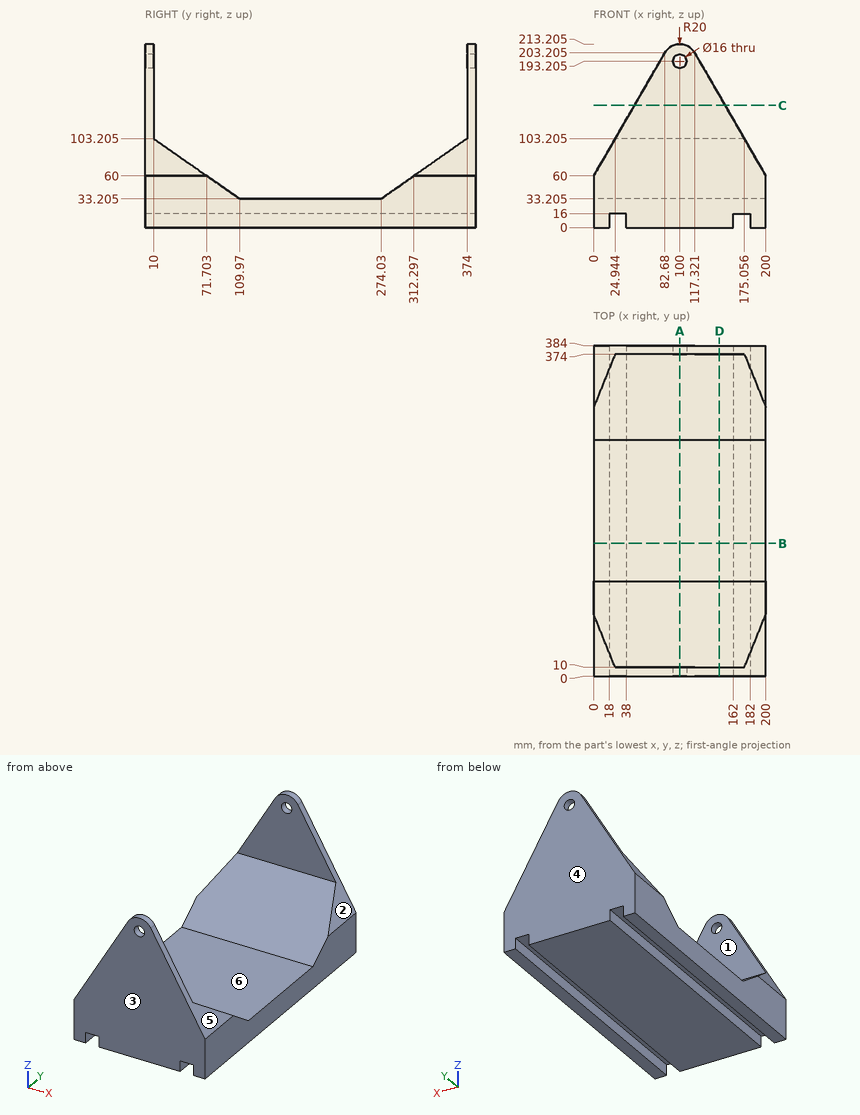
Study the drawing (mm; zero at the part's minimum x, y, z) and answer. A direction names the side the tool comes from. Give positions to 0.01 mm unless a question says otherwise; leave off trailing zeros. Write each loop counter-clockwise with the first axis right and the second up, starting at its lowest first coordinate (ties: lowest second). Pieces come first, ordered by that corner, then holes. Notation, with made-up numbers: (2, -10.75) - (61, -10.75) arc R26 ccw to (61, 6.25) - close; hole circle Ø6 at (80, 47). An arc over 180 degrees is marked (long way). Write item = value, one per line. Start each with the question number.
Item 1: Find the intervals of material crossed by probe 1 along Y at (x, z) = (119, 156.5); probe 2 along Z at (x, y) = (39, 228) (1 decimal); probe 3 along Y at (x, z) = (64, 35) (1 decimal), in increasing order. Write a range as [from, to].
Item 2: Find section D-D (x = 146). Give the vertices of the cut face in (y, z) (1 decimal).
Item 3: Find section B-B (y = 154). Give the vertices of the cut face in (x, z) (1 decimal), then the cut area to 3 significant figures.
Item 4: A tool of negligible diameter and unlimited length cuts with its end or side. For the marked faces 1 and 2, from which of +Z, -Z, +X, -X, +Y, -Y can it reach the whole face along a straight path? Write none if from no direction.
Item 5: Find section C-C (z = 142). Give the vertices of the cut face in (x, y).
Item 6: The mould has two halves that part along Y. Classify the marked faces 3, 4, 5 and 6: +Y half, -Y half, draft (parallel to the pull), parting line (faces both ways), or undercut.
Item 7: Each of these flat-tipped pins is pushed along its axis until it touches: P1, Ø3, axis at x = 86.5, y = 153, coming from the -Z side; P2, Ø8, axis at x = 161, y = 45.5, coming from the +Z side; P3, Ø13, axis at x = 100, z = 193.21, coming from the -Y side; P4, Ø6, axis at x = 168.5, y = 128, coming from the -Z side. Where does it stop, or does it pass through?
Item 8: Find section A-A (x = 100). Give the vertices of the cut face in (y, z) (1 decimal).
Response:
q1.probe_1 = [0, 10], [374, 384]
q1.probe_2 = [0, 33.2]
q1.probe_3 = [0, 107.4], [276.6, 384]
q2.outline = (0, 0) - (384, 0) - (384, 153.5) - (374, 153.5) - (374, 103.2) - (274, 33.2) - (110, 33.2) - (10, 103.2) - (10, 153.5) - (0, 153.5) - close
q3.outline = (0, 0) - (18, 0) - (18, 16) - (38, 16) - (38, 0) - (162, 0) - (162, 16) - (182, 16) - (182, 0) - (200, 0) - (200, 33.2) - (0, 33.2) - close
q3.area = 6,000 mm²
q4.face_1 = +Z, +X, -X
q4.face_2 = +Z, +X, +Y, -Y
q5.outline = (47.34, 0) - (152.66, 0) - (152.66, 10) - (47.34, 10) - close; (47.34, 374) - (152.66, 374) - (152.66, 384) - (47.34, 384) - close
q6.face_3 = -Y half
q6.face_4 = +Y half
q6.face_5 = draft
q6.face_6 = undercut
q7.P1 = 0
q7.P2 = 81.15
q7.P3 = through
q7.P4 = 16
q8.outline = (0, 0) - (384, 0) - (384, 185.2) - (374, 185.2) - (374, 103.2) - (274, 33.2) - (110, 33.2) - (10, 103.2) - (10, 185.2) - (0, 185.2) - close; (0, 201.2) - (10, 201.2) - (10, 213.2) - (0, 213.2) - close; (374, 201.2) - (384, 201.2) - (384, 213.2) - (374, 213.2) - close
